Could you check a few things on this model? Use its own coordinates, in mm. A direction names the side the tool comes from. Give positions to 0.01 mm unless a question says otherwise; leave off trailing zeros. Write each loop counter-clockwise with the first axis right and the second up, starting at its lowest first coordinate (ties: lowest second). Pieces come first, ordered by that corner, then holes. Notation, with made-up numbers: (28, 78) - (46, 78) arc R14 cw to (46, 95) - close; hole circle Ø1 at (-28.75, -25). An arc over 180 degrees is marked (long way). Answer as CSV lines item,"result". Start each with the question number.
Q1. On a 3-axis mill with a long thin cutter (end or side, diameter ignored), from which of +Z, -Z, +X, -X, +Y, -Y can I reach the whole of each face in a straight line? I mean faces 1 (the face through (-29.957, -12.661, -22.97)), 2 (the face through (8, -9.144, -8)), 3 (the face through (-35, 0, -16)). Say none if no direction works.
Q2. Imagine slicing it at A-A on x = 0. List the corners of the cut face in (y, z) for me.
Q3. Imagine slicing it at D-D on x = -42. List the corners of the cut face in (y, z) for me, and give its area (3 significant figures).
Q4. Will these pins go through, and if not, where does the flat tip stop? pin 1 Ø5 at (y, z) = (-12, -45.5) entering from -X; pin 2 Ø1.5 at (y, z) = (-10, -54) entering from +X; pin 3 Ø10 at (x, z) = (-15, -57) entering from +Y; pin 4 Ø6 at (y, z) = (-7.5, 18.5) entering from -X.
Q5. Imagine slicing it at C-C on z = -41.5. List the corners of the cut face in (x, y) for me, and give its area (3 significant figures).
Q6. We'd pull the mould along Z, two halves only. Please class faces 4 (the face through (72, -3, 23)), 5 (the face through (8, -15.494, -8)), 6 (the face through (-8.11, -6.67, -36.51)): pulls with the +Z half, pulls with the -Z half, needs draft (parallel to the pull), parting line crosses it, or undercut.
Q7. If I drill on line 1 along Z through (x, y) = (0, -3.25); line 2 along Y through (x, z) = (-14.5, -44); line 3 along Y through (x, z) = (-47.5, 51), over which ranges is the centre line in solid material (lowest first)?
Q8. Imagine slicing it at B-B on y = -3. List the corners of the cut face in (x, z) for me, and give its area (3 significant figures).
```python
from build123d import *

# Parameters (mm, degrees)
F0_R     = 75.5827918499
F0_R_2   = 61.792299123
F1_DEPTH = 5.08
F0_R_3   = 37.749771155
F2_DEPTH = 9.906
F0_R_4   = 10.2931337437
F3_DEPTH = 15.494
F4_DEPTH = 9.906
F5_DEPTH = 9.144
F5_TAPER = 3


with BuildPart() as f1:
    # F0 (on Front) → F1 (new body)
    with BuildSketch(Plane.XZ):
        Circle(F0_R)
        Circle(F0_R_2, mode=Mode.SUBTRACT)
    extrude(amount=F1_DEPTH)

    # F0 (on Front) → F2 (join)
    with BuildSketch(Plane.XZ):
        Circle(F0_R_2)
        Circle(F0_R_3, mode=Mode.SUBTRACT)
    extrude(amount=F2_DEPTH)

    # F0 (on Front) → F3 (join)
    with BuildSketch(Plane.XZ):
        Circle(F0_R_3)
        Circle(F0_R_4, mode=Mode.SUBTRACT)
    extrude(amount=F3_DEPTH)

    # F0 (on Front) → F4 (join)
    with BuildSketch(Plane.XZ):
        Circle(F0_R_3)
        Circle(F0_R_4, mode=Mode.SUBTRACT)
    extrude(amount=F4_DEPTH)

    # F0 (on Front) → F5 (cut)
    with BuildSketch(Plane.XZ):
        Circle(F0_R_3)
        Circle(F0_R_4, mode=Mode.SUBTRACT)
    extrude(amount=F5_DEPTH, taper=F5_TAPER, mode=Mode.SUBTRACT)


solid = f1.part
```
Conclusion:
1,face 1,"-Y"
1,face 2,"+Y"
1,face 3,"+Z, -Z, +X, -X, +Y"
2,outline,"(-15.49, -37.75) - (-9.91, -37.75) - (-9.91, -61.79) - (-5.08, -61.79) - (-5.08, -75.58) - (0, -75.58) - (0, -37.75) - (-9.14, -37.27) - (-9.14, -10.77) - (0, -10.29) - (-15.49, -10.29) - close; (-15.49, 10.29) - (0, 10.29) - (-9.14, 10.77) - (-9.14, 37.27) - (0, 37.75) - (0, 75.58) - (-5.08, 75.58) - (-5.08, 61.79) - (-9.91, 61.79) - (-9.91, 37.75) - (-15.49, 37.75) - close"
3,outline,"(-9.91, -45.32) - (-5.08, -45.32) - (-5.08, -62.84) - (0, -62.84) - (0, 62.84) - (-5.08, 62.84) - (-5.08, 45.32) - (-9.91, 45.32) - close"
3,area,"1,080 mm^2"
4,pin 1,"x = -43.25"
4,pin 2,"x = 31.34"
4,pin 3,"y = 0"
4,pin 4,"x = -73.71"
5,outline,"(-63.17, -5.08) - (-45.78, -5.08) - (-45.78, -9.91) - (45.78, -9.91) - (45.78, -5.08) - (63.17, -5.08) - (63.17, 0) - (-63.17, 0) - close"
5,area,"1,080 mm^2"
6,face 4,"parting line crosses it"
6,face 5,"needs draft"
6,face 6,"undercut"
7,line 1,"-75.58 to -37.58, -10.46 to -10.29, 10.29 to 10.46, 37.58 to 75.58"
7,line 2,"-9.91 to 0"
7,line 3,"-5.08 to 0"
8,outline,"circle Ø151.17 at (0, 0); circle Ø20.9 at (0, 0); hole circle Ø75.19 at (0, 0); hole circle Ø20.59 at (0, 0)"
8,area,"13,500 mm^2"
